```python
from build123d import *

# Parameters (mm, degrees)
SKETCH1_R           = 2
BOSS_EXTRUDE1_DEPTH = 8
SKETCH2_R           = 3.5
BOSS_EXTRUDE2_DEPTH = 2.5
SKETCH3_R           = 12.25
BOSS_EXTRUDE3_DEPTH = 53.8
SKETCH4_R           = 1.27
CUT_EXTRUDE1_DEPTH  = 0.254
SKETCH5_R           = 11.5
BOSS_EXTRUDE4_DEPTH = 16
CUT_EXTRUDE2_DEPTH  = 8


with BuildPart() as part:
    # Sketch1 → Boss-Extrude1 (new body)
    with BuildSketch(Plane.XY):
        Circle(SKETCH1_R)
    extrude(amount=BOSS_EXTRUDE1_DEPTH)

    # Sketch2 → Boss-Extrude2 (add)
    with BuildSketch(Plane(origin=(0, 0, 0), x_dir=(-1, 0, 0), z_dir=(0, 0, -1))):
        Circle(SKETCH2_R)
    extrude(amount=BOSS_EXTRUDE2_DEPTH)

    # Sketch3 → Boss-Extrude3 (add)
    with BuildSketch(Plane(origin=(0, 0, -2.5), x_dir=(-1, 0, 0), z_dir=(0, 0, -1))):
        Circle(SKETCH3_R)
    extrude(amount=BOSS_EXTRUDE3_DEPTH)

    # Sketch4 → Cut-Extrude1 (cut)
    with BuildSketch(Plane.XY.offset(-2.5)):
        with Locations((8.5, 0)):
            Circle(SKETCH4_R)
        with Locations((-8.5, 0)):
            Circle(SKETCH4_R)
    extrude(amount=-CUT_EXTRUDE1_DEPTH, mode=Mode.SUBTRACT)

    # Sketch5 → Boss-Extrude4 (add)
    with BuildSketch(Plane(origin=(0, 0, -56.3), x_dir=(-1, 0, 0), z_dir=(0, 0, -1))):
        Circle(SKETCH5_R)
    extrude(amount=BOSS_EXTRUDE4_DEPTH)

    # Sketch6 → Cut-Extrude2 (cut)
    with BuildSketch(Plane.XY.offset(8)):
        with BuildLine():
            Line((-1.322875656, 1.5), (1.322875656, 1.5))
            ThreePointArc((1.322875656, 1.5), (0, 2), (-1.322875656, 1.5))
        make_face()
    extrude(amount=-CUT_EXTRUDE2_DEPTH, mode=Mode.SUBTRACT)


solid = part.part
```
Here's how the part is built. I have some questions about the finished solid (model axes, mm). A direction names the side the tool comes from. Coordinates: 2 decimals unless noted, no trailing zeros. Order: outer loops, then holes, each group sorted by start corner. A loop starts at its lowest first (then second) coordinate and runs counter-clockwise, first axis right, second up.
Item 1: If we section it at C-C, the plane z = -31.5: List the corners of the cut face in (x, y) for me, then the cut area to 3 significant figures.
Response values:
outline: circle Ø24.5 at (0, 0)
area: 471 mm2
Item 2: If we section it at A-A, the plane y = 0: List the corners of the cut face in (x, z) for me.
Response values:
outline: (-12.25, -56.3) - (-11.5, -56.3) - (-11.5, -72.3) - (11.5, -72.3) - (11.5, -56.3) - (12.25, -56.3) - (12.25, -2.5) - (9.77, -2.5) - (9.77, -2.75) - (7.23, -2.75) - (7.23, -2.5) - (3.5, -2.5) - (3.5, 0) - (2, 0) - (2, 8) - (-2, 8) - (-2, 0) - (-3.5, 0) - (-3.5, -2.5) - (-7.23, -2.5) - (-7.23, -2.75) - (-9.77, -2.75) - (-9.77, -2.5) - (-12.25, -2.5) - close
Item 3: If we section it at B-B, the plane x = 0: List the corners of the cut face in (y, z) for me, then the cut area to 3 significant figures.
Response values:
outline: (-12.25, -56.3) - (-11.5, -56.3) - (-11.5, -72.3) - (11.5, -72.3) - (11.5, -56.3) - (12.25, -56.3) - (12.25, -2.5) - (3.5, -2.5) - (3.5, 0) - (1.5, 0) - (1.5, 8) - (-2, 8) - (-2, 0) - (-3.5, 0) - (-3.5, -2.5) - (-12.25, -2.5) - close
area: 1,730 mm2
Item 4: If we section it at D-D, the plane x = -6.25: List the corners of the cut face in (y, z) for me.
Response values:
outline: (-10.54, -56.3) - (-9.65, -56.3) - (-9.65, -72.3) - (9.65, -72.3) - (9.65, -56.3) - (10.54, -56.3) - (10.54, -2.5) - (-10.54, -2.5) - close
Item 5: I'm going to push flat-ended pins straight in: pin 1 Ø10 at (x, z) = (6.5, -52) entering from -Y; pin 2 Ø2 at (x, y) = (-8.5, 0) entering from +Z; pin 3 Ø1.3 at (x, z) = (0.5, 4) entering from +Y. Where does each tip first touch, or does it pass through?
Response values:
pin 1: stops at y = -12.16
pin 2: stops at z = -2.75
pin 3: stops at y = 1.5
Item 6: Which directions (+Z, -Z, +X, -X, +Y, -Y) give clear straight access to the entire face, cutting with the end or side of a thin tool? Please do faces 4 (the face through (0, 0, -72.3)), 5 (the face through (1.5, 11.4, -64.2)), 6 (the face through (0, 1.5, 4)), 7 (the face through (-3.233, -1.341, -1.232)), 8 (the face through (0, 0, 8)).
Response values:
face 4: -Z, +X, -X, +Y, -Y
face 5: -Z
face 6: +Z, +X, -X, +Y
face 7: +Z
face 8: +Z, +X, -X, +Y, -Y
Item 7: I need wall thicknesses on probe 1 along Z at (x, y) = (-7, 6.5); probe 2 along Y at (x, z) = (-8.5, -2.6); probe 3 along Z at (x, y) = (9.25, 0.75). Which ranges of each line are inside material? Lowest first, please.
Response values:
probe 1: z = -72.3 to -2.5
probe 2: y = -8.82 to -1.27, 1.27 to 8.82
probe 3: z = -72.3 to -2.75
Item 8: Thinking about a two-plate mould opening in Y: for faces 1 (the face through (11, -4, -56.3)), 2 (the face through (0, -2, 4)), 3 (the face through (8, 0, -2.754)), which applies, pulls with the +Y half, pulls with the -Y half, needs draft (parallel to the pull), parting line crosses it, or undercut?
Response values:
face 1: needs draft
face 2: parting line crosses it
face 3: undercut
